Can you work these out from the model? Positions are in its coordinate system, mm. Coordinates: 2 decimals unless noted, no trailing zeros. Order: outer loops, then holes, each group sorted by start corner. A loop starts at its lowest first (then second) coordinate and runs counter-clockwise, first axis right, second up.
```python
from build123d import *

# Parameters (mm, degrees)
SKETCH1_R             = 45.72
BOSS_EXTRUDE1_DEPTH   = 9.525
SKETCH2_R             = 14.3002
CUT_EXTRUDE1_DEPTH    = 10.525
F_8_CLEARANCE_HOLE1_D = 4.4958
CIRPATTERN1_COUNT     = 6


with BuildPart() as part:
    # Sketch1 → Boss-Extrude1 (new body)
    with BuildSketch(Plane(origin=(0, 0, 0), x_dir=(0, 0, -1), z_dir=(1, 0, 0))):
        Circle(SKETCH1_R)
    extrude(amount=BOSS_EXTRUDE1_DEPTH)

    # Sketch2 → Cut-Extrude1 (cut, through all)
    with BuildSketch(Plane.ZY):
        Circle(SKETCH2_R)
    extrude(amount=-CUT_EXTRUDE1_DEPTH, mode=Mode.SUBTRACT)

    # #8 Clearance Hole1 (through all)
    with Locations(Plane.ZY):
        with Locations((0, 23.8125)):
            f_8_clearance_hole1 = Hole(F_8_CLEARANCE_HOLE1_D / 2)

    # CirPattern1: #8 Clearance Hole1 ×6 about axis
    cirpattern1_axis = Axis((0, 0, 0), (1, 0, 0))
    for i in range(1, CIRPATTERN1_COUNT):
        add(f_8_clearance_hole1.rotate(cirpattern1_axis, i * 360 / CIRPATTERN1_COUNT), mode=Mode.SUBTRACT)


solid = part.part
```
1. Please list where these lines run through material, in increasing order: probe 1 along Y at (x, z) = (5.5, 0); probe 2 along Z at (x, y) = (7.5, -10); probe 3 along Z at (x, y) = (4.75, -11).
Completed:
probe 1: y = -45.72 to -26.06, -21.56 to -14.3, 14.3 to 21.56, 26.06 to 45.72
probe 2: z = -44.61 to -21.81, -19.43 to -10.22, 10.22 to 19.43, 21.81 to 44.61
probe 3: z = -44.38 to -22.68, -18.57 to -9.14, 9.14 to 18.57, 22.68 to 44.38
2. Thinking about a two-plate mould opening in Y: for faces 1 (the cylindrical face through (4.7, -13.96, -3.1)), 2 (the cylindrical face through (4.7, 13.73, -43.61)), 3 (the cylindrical face through (4.829, 25.708, -1.208)), 4 (the flat face through (0, -10, 11)), which applies, pulls with the +Y half, pulls with the -Y half, needs draft (parallel to the pull), parting line crosses it, or undercut?
Completed:
face 1: undercut
face 2: parting line crosses it
face 3: undercut
face 4: needs draft
3. Imagine slicing it at B-B on z = 0. Please give me the cut outline in (x, y) (3 decimals), then the cut area to 3 significant figures.
Completed:
outline: (0, -45.72) - (9.525, -45.72) - (9.525, -26.06) - (0, -26.06) - close; (0, -21.565) - (9.525, -21.565) - (9.525, -14.3) - (0, -14.3) - close; (0, 14.3) - (9.525, 14.3) - (9.525, 21.565) - (0, 21.565) - close; (0, 26.06) - (9.525, 26.06) - (9.525, 45.72) - (0, 45.72) - close
area: 513 mm2
4. Imagine slicing it at D-D on z = -40. Please give me the cut outline in (x, y) (3 decimals).
Completed:
outline: (0, -22.143) - (9.525, -22.143) - (9.525, 22.143) - (0, 22.143) - close
5. Imagine slicing it at C-C on x = 3. Please give me the cut outline in (y, z).
Completed:
outline: circle Ø91.44 at (0, 0); hole circle Ø4.5 at (-23.81, 0); hole circle Ø28.6 at (0, 0); hole circle Ø4.5 at (-11.91, -20.62); hole circle Ø4.5 at (-11.91, 20.62); hole circle Ø4.5 at (11.91, -20.62); hole circle Ø4.5 at (11.91, 20.62); hole circle Ø4.5 at (23.81, 0)
6. Imagine slicing it at A-A on y = 0. Please give me the cut outline in (x, z) (3 decimals).
Completed:
outline: (0, -45.72) - (9.525, -45.72) - (9.525, -14.3) - (0, -14.3) - close; (0, 14.3) - (9.525, 14.3) - (9.525, 45.72) - (0, 45.72) - close
7. I'm going to push flat-ended pins straight in: pin 1 (1 mm diameter, centred on x = 5.5, y = -1, fed in from +Z); pin 2 (3.5 mm diameter, centred on y = 23.81, z = 0, fed in from -X); pin 3 (1 mm diameter, centred on x = 1, y = -16.5, fed in from -Z); pin 4 (2 mm diameter, centred on x = 1.5, y = 14, fed in from -Z). Where does each tip first touch, or does it pass through?
Completed:
pin 1: stops at z = 45.72
pin 2: passes through
pin 3: stops at z = -42.83
pin 4: stops at z = -43.83
